from build123d import *

# Parameters (mm, degrees)
SKETCH1_W           = 79.375
SKETCH1_H           = 79.375
BOSS_EXTRUDE1_DEPTH = 4
SKETCH2_R           = 11.90625
BOSS_EXTRUDE2_DEPTH = 8
SKETCH3_R           = 1.7859375
CUT_EXTRUDE1_DEPTH  = 12


with BuildPart() as part:
    # Sketch1 → Boss-Extrude1 (new body)
    with BuildSketch(Plane(origin=(0, 0, 0), x_dir=(1, 0, 0), z_dir=(0, 1, 0))):
        with Locations((39.6875, 39.6875)):
            Rectangle(SKETCH1_W, SKETCH1_H)
    extrude(amount=BOSS_EXTRUDE1_DEPTH)

    # Sketch2 → Boss-Extrude2 (add)
    with BuildSketch(Plane(origin=(0, 4, 0), x_dir=(1, 0, 0), z_dir=(0, 1, 0))):
        with Locations((39.6875, 39.6875)):
            Circle(SKETCH2_R)
    extrude(amount=BOSS_EXTRUDE2_DEPTH)

    # Sketch3 → Cut-Extrude1 (cut)
    with BuildSketch(Plane(origin=(0, 12, 0), x_dir=(1, 0, 0), z_dir=(0, 1, 0))):
        with Locations((34.7265625, 39.6875)):
            Circle(SKETCH3_R)
        with Locations((44.6484375, 39.6875)):
            Circle(SKETCH3_R)
    extrude(amount=-CUT_EXTRUDE1_DEPTH, mode=Mode.SUBTRACT)


solid = part.part
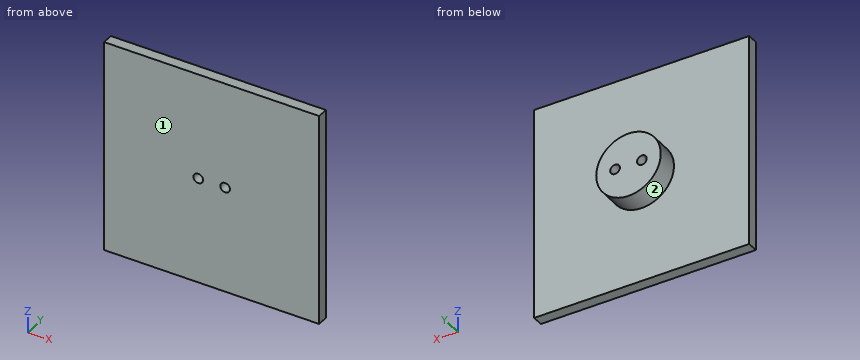
Geometry: final body of the model. Coordinates: model frame, mm. Face numbers are marked on the shaded views. A direction names the side the tool comes from. Round coordinates to 2 decimals unless told otherwise and drop trailing zeros. Order: outer loops, then holes, each group sorted by start corner. A loop starts at its lowest first (then second) coordinate and runs counter-clockwise, first axis right, second up. Notation, with made-up numbers: (63, 56.25) -> (95, 56.25) arc R13 ccw to (95, 70.25) -> close; hole circle Ø4 at (20.5, 43.25). An arc over 180 degrees is marked (long way). Put each result on its own line as item: value. Start each with the question number.
Q1. Section C-C on z = -23. Return the cut outline in (x, y) (3 decimals).
Q2. First-contact query: pin 1 (5 mm diameter, centred on y = 8, z = -50.5, fed in from -X); pin 2 (1.5 mm diameter, centred on y = 7.5, z = -40.5, fed in from +X). Flat tips, straight axial feed; report the tip coordinate or a pass-through.
Q3. Reachability of the marked faces 1 and 2 from +Z, -Z, +X, -X, +Y, -Y: full face, straight path, thin tool, end or side. Return the list, or none.
Q4. Section A-A on x = 35.5. Return the cut outline in (y, z) (3 decimals), and give its area (3 significant figures).
Q5. Section D-D on y = 6.75. Return the cut outline in (x, z).
Q6. Line query: probe 1 along Y at (x, z) = (31, -60); probe 2 along Z at (x, y) = (44.5, 9.5); probe 3 along Z at (x, y) = (41, 4.25). Output: solid intervals per line, ascending.
Q7. Section B-B on x = 72. Return the cut outline in (y, z) (3 decimals), and give its area (4 significant figures).
Ans:
1. outline: (0, 0) -> (79.375, 0) -> (79.375, 4) -> (0, 4) -> close
2. pin 1: stops at x = 31.16
2. pin 2: stops at x = 51.59
3. face 1: +Z, -Z, +X, -X, -Y
3. face 2: +Y
4. outline: (0, -79.375) -> (4, -79.375) -> (4, -50.833) -> (12, -50.833) -> (12, -41.297) -> (0, -41.297) -> close; (0, -38.078) -> (12, -38.078) -> (12, -28.542) -> (4, -28.542) -> (4, 0) -> (0, 0) -> close
4. area: 457 mm2
5. outline: circle Ø23.81 at (39.69, -39.69); hole circle Ø3.57 at (34.73, -39.69); hole circle Ø3.57 at (44.65, -39.69)
6. probe 1: y = 0 to 4
6. probe 2: z = -50.58 to -41.47, -37.91 to -28.8
6. probe 3: z = -51.52 to -27.85
7. outline: (0, -79.375) -> (4, -79.375) -> (4, 0) -> (0, 0) -> close
7. area: 317.5 mm2
